Autodesk Inventor part; units mm, degrees
ref_plane "YZ Plane" through (0, 0, 0) normal (1, 0, 0) x (0, 1, 0)
ref_plane "XZ Plane" through (0, 0, 0) normal (0, 1, 0) x (-1, 0, 0)
ref_plane "XY Plane" through (0, 0, 0) normal (0, 0, 1) x (1, 0, 0)
sketch "Boceto1" plane through (0, 0, 0) normal (0, 0, 1) x (1, 0, 0)
  line L0 (5, 0) -> (30, 0)
  line L1 (35, 5) -> (35, 60)
  line L2 (30, 65) -> (5, 65)
  line L3 (0, 60) -> (0, 5)
  arc A0 (5, 65) -> (0, 60) centre (5, 60) ccw
  arc A1 (35, 60) -> (30, 65) centre (30, 60) ccw
  arc A2 (0, 5) -> (5, 0) centre (5, 5) ccw
  arc A3 (30, 0) -> (35, 5) centre (30, 5) ccw
  circle A4 centre (17.5, 55) radius 2.5
  circle A5 centre (5, 8.75) radius 2.5
  circle A6 centre (30, 8.75) radius 2.5
  point P0 (0, 0)
extrude "Extrusión1" add sketch "Boceto1" along normal blind 3
properties part number "6"
Input: part model. Units: mm. Frame: model coordinates. Coordinates: 2 decimals unless noted, no trailing zeros. Loops run counter-clockwise (first coordinate to the right, second up) from the corner with the lowest first, then second, coordinate; pieces in that order, holes last. Notation, with made-up numbers: (29.25, 59.5) - (51.25, 59.5) arc R22 ccw to (51.25, 88.5) - close; hole circle Ø7 at (-22, 89). An arc over 180 degrees is marked (long way). Answer in a Markdown table with one row per item. Add a question column.
Item 1: Section query A-A on y = 55. Return the cut outline in (x, z), then the cut area to 3 significant figures.
Item 2: Mould query, pull axis Y, two halves, no side actions, for faces 1 (the cylindrical face through (29.5, 11.2, 1.5)), 2 (the cylindrical face through (6.15, 10.97, 1.48)), 3 (the cylindrical face through (34, 2, 1)), 4 (the cylindrical face through (33, 64, 1)). Classes: released by +Y, released by -Y, zero draft, split by the parting line, or undercut.
Item 3: Section query C-C on x = 31.5. Return the cut outline in (y, z), then the cut area to 3 significant figures.
Item 4: Line query: line 1 along Y through (x, z) = (17.5, 1.5); line 2 along Y through (x, z) = (5, 1.05); line 3 along X through (y, z) = (10.5, 1.7). Output: solid intervals per line, ascending. Write a range as [from, to].
Item 5: Section query B-B on z = 2.2. Return the cut outline in (x, y).
Recorded:
| question | item | result |
|---|---|---|
| 1 | outline | (0, 0) - (15, 0) - (15, 3) - (0, 3) - close; (20, 0) - (35, 0) - (35, 3) - (20, 3) - close |
| 1 | area | 90.0 mm^2 |
| 2 | face 1 | undercut |
| 2 | face 2 | undercut |
| 2 | face 3 | released by -Y |
| 2 | face 4 | released by +Y |
| 3 | outline | (0.23, 0) - (6.75, 0) - (6.75, 3) - (0.23, 3) - close; (10.75, 0) - (64.77, 0) - (64.77, 3) - (10.75, 3) - close |
| 3 | area | 182 mm^2 |
| 4 | line 1 | [0, 52.5], [57.5, 65] |
| 4 | line 2 | [0, 6.25], [11.25, 65] |
| 4 | line 3 | [0, 3.21], [6.79, 28.21], [31.79, 35] |
| 5 | outline | (0, 5) arc R5 ccw to (5, 0) - (30, 0) arc R5 ccw to (35, 5) - (35, 60) arc R5 ccw to (30, 65) - (5, 65) arc R5 ccw to (0, 60) - close; hole circle Ø5 at (5, 8.75); hole circle Ø5 at (17.5, 55); hole circle Ø5 at (30, 8.75) |
